The listing builds one solid part. Answer for the finished solid, in the listing's coordinates (mm). Coordinates: 2 decimals unless noted, no trailing zeros. Order: outer loops, then holes, each group sorted by start corner. A loop starts at its lowest first (then second) coordinate and runs counter-clockwise, first axis right, second up. Notation, with made-up numbers: (11.5, 68) -> (28.5, 68) arc R28 ccw to (28.5, 97) -> close; hole circle Ø3 at (80.5, 39.25). An arc over 180 degrees is marked (long way). Answer in a Markdown table with one row per item.
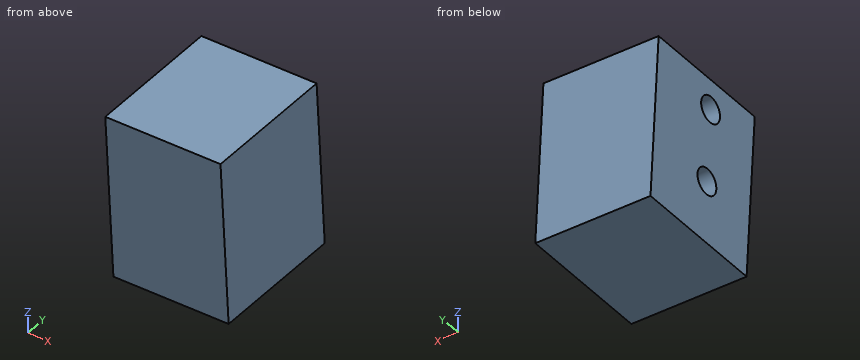
```python
from build123d import *

# Parameters (mm, degrees)
BOSS_EXTRUDE1_DEPTH         = 40
M10X1_25_TAPPED_HOLE1_D     = 8.8
M10X1_25_TAPPED_HOLE1_DEPTH = 10
M10X1_25_TAPPED_HOLE1_TIP   = 2.643786724


with BuildPart() as part:
    # Sketch1 → Boss-Extrude1 (new body)
    with BuildSketch(Plane(origin=(-407.523949035, -1.773656994, -6.913182302), x_dir=(0.01696126662903347, 3.690723310511945e-05, -0.99985614668921), z_dir=(0.9998466777110684, 0.004351609412378134, 0.016961266629033474))):
        Polygon((-575.226758447, 44.985593464), (-573.177194833, 0.028597337), (-517.605829152, 2.562063958), (-519.655392766, 47.519060086), align=None)
    extrude(amount=BOSS_EXTRUDE1_DEPTH)

    # M10x1.25 Tapped Hole1
    with Locations(Plane(origin=(-407.523949035, -1.773656994, -6.913182302), x_dir=(-0.016961266629033415, -3.690723310511849e-05, 0.99985614668921), z_dir=(-0.9998466777110684, -0.004351609412377967, -0.016961266629033418))):
        with Locations((564.098413091, 20.463266947), (539.12435261, 21.601820011)):
            Hole(M10X1_25_TAPPED_HOLE1_D / 2, depth=M10X1_25_TAPPED_HOLE1_DEPTH)
            with Locations((0, 0, -(M10X1_25_TAPPED_HOLE1_DEPTH + M10X1_25_TAPPED_HOLE1_TIP / 2))):  # 118° drill point
                Cone(0, M10X1_25_TAPPED_HOLE1_D / 2, M10X1_25_TAPPED_HOLE1_TIP, mode=Mode.SUBTRACT)


solid = part.part
```
(1) Find the intervals of material crossed by line 1 along Y through (x, z) = (-407.5, 534); line 2 along Y through (x, z) = (-396.5, 528); line 3 along Z through (x, y) = (-401.5, 12), in increasing order. Write a range as from..to.
Check values:
| item | result |
|---|---|
| line 1 | -0.25..15.79, 23.9..44.8 |
| line 2 | 0.08..45.13 |
| line 3 | 511.38..567.07 |
(2) Flat-ended cylindrical pins translate along their axes: pin 1 (1.5 mm diameter, centred on x = -405.5, y = 28, fed in from +Z); pin 2 (5 mm diameter, centred on x = -387, y = 4.5, fed in from -Z); pin 3 (2 mm diameter, centred on y = 32, z = 543, fed in from -X). Find the tip coordinate at first contact, or state that the pin passes through.
Check values:
| item | result |
|---|---|
| pin 1 | z = 567.77 |
| pin 2 | z = 511.16 |
| pin 3 | x = -417.02 |
(3) A cutting plane is placed at C-C, the plane x = -406. Count the separate pieces of the cut face and the enclosed holes in it, then the cut area to 3 significant figures.
Check values:
| item | result |
|---|---|
| separate pieces | 1 |
| enclosed holes | 2 |
| area | 2,450 mm² |
(4) A cutting plane is placed at B-B, the plane x = -388.5. Determine the outline of the cut face in (y, z), then the cut area to 3 significant figures.
Check values:
| item | result |
|---|---|
| outline | (-1.64, 566.67) -> (0.89, 511.09) -> (45.85, 513.14) -> (43.32, 568.72) -> close |
| area | 2,500 mm² |
(5) A cutting plane is placed at A-A, the plane z = 521.5. Determine the outline of the cut face in (x, y).
Check values:
| item | result |
|---|---|
| outline | (-416.69, 45.32) -> (-416.5, 0.27) -> (-376.49, 0.48) -> (-376.69, 45.53) -> close |
